from build123d import *

# Parameters (mm, degrees)
SKETCH1_W           = 101.6
SKETCH1_H           = 101.6
BOSS_EXTRUDE1_DEPTH = 10
SKETCH2_R           = 5
CUT_EXTRUDE1_DEPTH  = 5
SKETCH3_R           = 12.5
BOSS_EXTRUDE2_DEPTH = 2
SKETCH4_R           = 7.75
BOSS_EXTRUDE3_DEPTH = 45


with BuildPart() as part:
    # Sketch1 → Boss-Extrude1 (new body)
    with BuildSketch(Plane(origin=(0, 0, 0), x_dir=(1, 0, 0), z_dir=(0, 1, 0))):
        Rectangle(SKETCH1_W, SKETCH1_H)
    extrude(amount=BOSS_EXTRUDE1_DEPTH)

    # Sketch2 → Cut-Extrude1 (cut)
    with BuildSketch(Plane(origin=(0, 0, 0), x_dir=(-1, 0, 0), z_dir=(0, -1, 0))):
        with Locations(Location((0, 0, 0), (0, 0, 90))):
            Circle(SKETCH2_R)
    extrude(amount=-CUT_EXTRUDE1_DEPTH, mode=Mode.SUBTRACT)

    # Sketch3 → Boss-Extrude2 (add)
    with BuildSketch(Plane(origin=(0, 10, 0), x_dir=(1, 0, 0), z_dir=(0, 1, 0))):
        with Locations(Location((0, 0, 0), (0, 0, 90))):
            Circle(SKETCH3_R)
    extrude(amount=BOSS_EXTRUDE2_DEPTH)

    # Sketch4 → Boss-Extrude3 (add)
    with BuildSketch(Plane(origin=(0, 12, 0), x_dir=(1, 0, 0), z_dir=(0, 1, 0))):
        with Locations(Location((0, 0, 0), (0, 0, 90))):
            Circle(SKETCH4_R)
    extrude(amount=BOSS_EXTRUDE3_DEPTH)


solid = part.part
CAD build for the part. Positions are in the model's coordinates, mm. A direction names the side the tool comes from. Round coordinates to 2 decimals unless told otherwise and drop trailing zeros. Order: outer loops, then holes, each group sorted by start corner. A loop starts at its lowest first (then second) coordinate and runs counter-clockwise, first axis right, second up. Notation, with made-up numbers: (12, 39.25) -> (18, 39.25) arc R22 ccw to (18, 73.25) -> close; hole circle Ø4 at (58, -31). An arc over 180 degrees is marked (long way). Write item = value, one per line. Start each with the question number.
(1) Pin check, flat tips, straight feed: P1, Ø1.5, axis at x = -5.5, y = 49, coming from the -Z side; P2, Ø1, axis at x = 31.5, z = -12.5, coming from the +Y side; P3, Ø3, axis at x = -2, z = 0.5, coming from the -Y side. Stop position of each tip, or through.
(2) Pull direction Z, two halves, no side cores. Call faces 1 (the cylindrical face through (-3.755, 10.986, -11.923)), 2 (the flat face through (0, 57, 0)), 3 (the cylindrical face through (-4.88, 2.46, 1.08)): released by +Z, released by -Z, zero draft, split by the parting line, or undercut.
(3) Which spindle directions (+Z, -Z, +X, -X, +Y, -Y) get a long thin tool onto all of the face, cutting with end or side? Do faces 4 (the flat face through (-1, 5, -50.8)), 5 (the cylindrical face through (-7.684, 34.185, 1.009)), 6 (the flat face through (0, 5, 0)). Say none if no direction does.
(4) Cut at B-B, the plane x = 0. List the corners of the cut face in (y, z).
(5) Cut at C-C, the plane y = 43.5. List the corners of the cut face in (x, z), then the cut area to 3 significant figures.
(6) Cut at A-A, the plane z = 0. List the corners of the cut face in (x, y).
(7) Probe line 1 (X direction, y = 1, z = 0); line 2 (Y direction, x = -3.5, z = -42); line 3 (Z direction, x = 4, y = 51). List the from-to ranges inside material, lowest first. Write a range as [from, to].
(8) Cut at D-D, the plane x = 41. List the corners of the cut face in (y, z).
Model answer:
q1.P1 = -6.12
q1.P2 = 10
q1.P3 = 5
q2.face_1 = split by the parting line
q2.face_2 = zero draft
q2.face_3 = undercut
q3.face_4 = -Z, +X, -X, +Y, -Y
q3.face_5 = +Y
q3.face_6 = -Y
q4.outline = (0, -50.8) -> (10, -50.8) -> (10, -12.5) -> (12, -12.5) -> (12, -7.75) -> (57, -7.75) -> (57, 7.75) -> (12, 7.75) -> (12, 12.5) -> (10, 12.5) -> (10, 50.8) -> (0, 50.8) -> (0, 5) -> (5, 5) -> (5, -5) -> (0, -5) -> close
q5.outline = circle Ø15.5 at (0, 0)
q5.area = 189 mm2
q6.outline = (-50.8, 0) -> (-5, 0) -> (-5, 5) -> (5, 5) -> (5, 0) -> (50.8, 0) -> (50.8, 10) -> (12.5, 10) -> (12.5, 12) -> (7.75, 12) -> (7.75, 57) -> (-7.75, 57) -> (-7.75, 12) -> (-12.5, 12) -> (-12.5, 10) -> (-50.8, 10) -> close
q7.line_1 = [-50.8, -5], [5, 50.8]
q7.line_2 = [0, 10]
q7.line_3 = [-6.64, 6.64]
q8.outline = (0, -50.8) -> (10, -50.8) -> (10, 50.8) -> (0, 50.8) -> close
